from build123d import *

# Parameters (mm, degrees)
EXTRUDE_DEPTH                     = 10.7
EXTRUDE_ONTO_SKETCH002_ROLL_ANGLE = 90
BOX021_W                          = 1.8
BOX021_H                          = 16
BOX021_DEPTH                      = 4
BOX_W                             = 38.34
BOX_H                             = 14
BOX_DEPTH                         = 2.5
BOX007_W                          = 55.2
BOX007_H                          = 2
BOX007_DEPTH                      = 27
BOX008_W                          = 2
BOX008_H                          = 16
BOX008_DEPTH                      = 27
BOX009_W                          = 1.8
BOX009_H                          = 16
BOX009_DEPTH                      = 4
BOX019_W                          = 13.4
BOX019_H                          = 14
BOX019_DEPTH                      = 1.2
BOX018_W                          = 38.34
BOX018_H                          = 14
BOX018_DEPTH                      = 2.5
BOX020_W                          = 55.2
BOX020_H                          = 14
BOX020_DEPTH                      = 1.4
BOX005_W                          = 13.4
BOX005_H                          = 14
BOX005_DEPTH                      = 1.2


with BuildPart() as motorclipholes:
    # Sketch002 as drawn → Extrude (new)
    with BuildSketch(Plane.XY):
        Polygon((16.24, -0.5), (18.24, -0.5), (18.24, -2.5), align=None)
        Polygon((18.24, 22.1), (18.24, 20.1), (16.24, 20.1), align=None)
    extrude(amount=-EXTRUDE_DEPTH)


with BuildPart() as motorclipholes_1:
    # Extrude onto Sketch002 roll: moved
    add(motorclipholes.part.rotate(Axis((0, 0, 0), (1, 0, 0)), EXTRUDE_ONTO_SKETCH002_ROLL_ANGLE))


with BuildPart() as motorclipholes_2:
    # Extrude onto Sketch002 placement: moved
    add(motorclipholes_1.part.moved(Location((-0.9, -37, 0))))


with BuildPart() as cube020:
    # Box021 → Box021 (new body)
    with BuildSketch(Plane(origin=(35.1, -37, 20), x_dir=(1, 0, 0), z_dir=(0, 0, 1))):
        with Locations((0.9, 8)):
            Rectangle(BOX021_W, BOX021_H)
    extrude(amount=BOX021_DEPTH)


with BuildPart() as cube003:
    # Box → Box (new body)
    with BuildSketch(Plane(origin=(-20.1, -37, -3), x_dir=(1, 0, 0), z_dir=(0, 0, 1))):
        with Locations((19.17, 7)):
            Rectangle(BOX_W, BOX_H)
    extrude(amount=BOX_DEPTH)


with BuildPart() as cube006:
    # Box007 → Box007 (new body)
    with BuildSketch(Plane(origin=(-20.1, -23, -3), x_dir=(1, 0, 0), z_dir=(0, 0, 1))):
        with Locations((27.6, 1)):
            Rectangle(BOX007_W, BOX007_H)
    extrude(amount=BOX007_DEPTH)


with BuildPart() as cube007:
    # Box008 → Box008 (new body)
    with BuildSketch(Plane(origin=(-22.1, -37, -3), x_dir=(1, 0, 0), z_dir=(0, 0, 1))):
        with Locations((1, 8)):
            Rectangle(BOX008_W, BOX008_H)
    extrude(amount=BOX008_DEPTH)


with BuildPart() as cube008:
    # Box009 → Box009 (new body)
    with BuildSketch(Plane(origin=(35.1, -37, -3), x_dir=(1, 0, 0), z_dir=(0, 0, 1))):
        with Locations((0.9, 8)):
            Rectangle(BOX009_W, BOX009_H)
    extrude(amount=BOX009_DEPTH)


with BuildPart() as cube018:
    # Box019 → Box019 (new body)
    with BuildSketch(Plane(origin=(21.7, -37, 21.4), x_dir=(1, 0, 0), z_dir=(0, 0, 1))):
        with Locations((6.7, 7)):
            Rectangle(BOX019_W, BOX019_H)
    extrude(amount=BOX019_DEPTH)


with BuildPart() as cube017:
    # Box018 → Box018 (new body)
    with BuildSketch(Plane(origin=(-20.1, -37, 20.1), x_dir=(1, 0, 0), z_dir=(0, 0, 1))):
        with Locations((19.17, 7)):
            Rectangle(BOX018_W, BOX018_H)
    extrude(amount=BOX018_DEPTH)


with BuildPart() as cube019:
    # Box020 → Box020 (new body)
    with BuildSketch(Plane(origin=(-20.1, -37, 22.6), x_dir=(1, 0, 0), z_dir=(0, 0, 1))):
        with Locations((27.6, 7)):
            Rectangle(BOX020_W, BOX020_H)
    extrude(amount=BOX020_DEPTH)


with BuildPart() as motorholder:
    # Box005 → Box005 (new body)
    with BuildSketch(Plane(origin=(21.7, -37, -3), x_dir=(1, 0, 0), z_dir=(0, 0, 1))):
        with Locations((6.7, 7)):
            Rectangle(BOX005_W, BOX005_H)
    extrude(amount=BOX005_DEPTH)

    # Fusion007: union Cube020, Cube003, Cube006, Cube007, Cube008, Cube018, Cube017, Cube019
    add(cube020.part)
    add(cube003.part)
    add(cube006.part)
    add(cube007.part)
    add(cube008.part)
    add(cube018.part)
    add(cube017.part)
    add(cube019.part)


with BuildPart() as motorholder_1:
    # Fusion007 placement: moved
    add(motorholder.part.moved(Location((-0.9, 0, 0))))

    # Cut017: cut motorClipHoles
    add(motorclipholes_2.part, mode=Mode.SUBTRACT)


with BuildPart() as mirror_of_motorholder:
    # mirror: instance of motorHolder
    add(motorholder_1.part.mirror(Plane(origin=(-23, -21, 0), x_dir=(-1, 0, 0), z_dir=(0, -1, 0))))


with BuildPart() as mirror_of_motorholder_1:
    # mirror placement: moved
    add(mirror_of_motorholder.part.moved(Location((0, 55, 0))))


solid = mirror_of_motorholder_1.part
Read the model definition and answer for the solid it produces. Units are mm, in the model's axes. A direction names the side the tool comes from. Round coordinates to 2 decimals unless told otherwise and drop trailing zeros. Order: outer loops, then holes, each group sorted by start corner. A loop starts at its lowest first (then second) coordinate and runs counter-clockwise, first axis right, second up.
1) Flat-ended cylindrical pins translate along their axes: pin 1 (6 mm diameter, centred on y = 39.5, z = 4.5, fed in from +X); pin 2 (0.6 mm diameter, centred on y = 34.5, z = 7.5, fed in from +X); pin 3 (5 mm diameter, centred on x = 3.5, z = 9, fed in from +Y). Find the tip coordinate at first contact, or state that the pin passes through.
2) The mould has two halves that part along X. Classify faces 5 (the face through (35, 42, 1)), 6 (the face through (34.2, 43, 0)), 7 (the face through (-23, 42, 10)): released by +X, released by -X, zero draft, split by the parting line, or undercut.
3) For faces 1 (the face through (34.2, 35, 10)), 2 (the face through (34.2, 43, 21)), 3 (the face through (30, 50, -2)), 4 (the face through (17.34, 38, -2)), determine the directions among +Z, -Z, +X, -X, +Y, -Y from which every point of the face is accessible in a straight line to the end or side of a thin tool.
4) Straight lines are drawn through the part: L1, parallel to Z at x = 11.5, y = 40.25; L2, parallel to X at y = 38.75, z = 22.25; L3, parallel to X at y = 43.75, z = 0.25. For each, find the intervals that lie inside material, in ascending order.
5) The part is cut by section C-C on z = 10.5. Write down the section's boundary in (x, y).
6) The part is cut by section B-B on x = 16. Write down the section's boundary in (y, z).
7) The part is cut by section D-D on x = -14. Write down the section's boundary in (y, z), plus the area to 3 significant figures.
8) The part is cut by section A-A on y = 43.25. Write down the section's boundary in (x, z).
Resolved:
1. pin 1: stops at x = -21
1. pin 2: stops at x = 34.2
1. pin 3: stops at y = 36
2. face 5: zero draft
2. face 6: undercut
2. face 7: released by -X
3. face 1: +X, +Y, -Y
3. face 2: +Y
3. face 3: +Z, -Z, +X, -X, +Y
3. face 4: -Z, +Y
4. L1: z = -3 to -0.5, 20.1 to 24
4. L2: x = -23 to 17.34, 20.8 to 36
4. L3: x = -23 to -21, 34.2 to 36
5. outline: (-23, 34) - (34.2, 34) - (34.2, 36) - (-21, 36) - (-21, 50) - (-23, 50) - close
6. outline: (34, -3) - (50, -3) - (50, -1.16) - (39.3, -1.16) - (39.3, -0.5) - (36, -0.5) - (36, 20.1) - (39.3, 20.1) - (39.3, 20.76) - (50, 20.76) - (50, 24) - (34, 24) - close
7. outline: (34, -3) - (50, -3) - (50, -0.5) - (36, -0.5) - (36, 20.1) - (50, 20.1) - (50, 24) - (34, 24) - close
7. area: 144 mm2
8. outline: (-23, -3) - (17.34, -3) - (17.34, -2.5) - (15.34, -0.5) - (-21, -0.5) - (-21, 20.1) - (15.34, 20.1) - (17.34, 22.1) - (17.34, 22.6) - (20.8, 22.6) - (20.8, 21.4) - (34.2, 21.4) - (34.2, 20) - (36, 20) - (36, 24) - (-23, 24) - close; (20.8, -3) - (36, -3) - (36, 1) - (34.2, 1) - (34.2, -1.8) - (20.8, -1.8) - close
